The listing builds one solid part. Answer for the finished solid, in the listing's coordinates (mm). A direction names the side the tool comes from. Round coordinates to 2 decimals unless told otherwise and drop trailing zeros. Order: outer loops, then holes, each group sorted by start corner. A loop starts at its lowest first (then second) coordinate and runs counter-clockwise, first axis right, second up. Notation, with made-up numbers: M 87,51.25 L 92,51.25 A26 ccw 92,76.25 Z; hole C -28.5,-6.5 d11. An arc over 180 degrees is marked long. Write item = value, one per line. Start each with the question number.
(1) A cutting plane is placed at B-B, the plane y = 6.75. Determine the outline of the cut face in (x, z), and give its area (3 significant figures).
(2) A cutting plane is placed at C-C, the plane x = 0. Determine the outline of the cut face in (y, z).
(3) A cutting plane is placed at A-A, the plane x = 130. Determine the outline of the cut face in (y, z), and give its area (3 significant figures).
(4) Straight lines are drawn through the part: probe 1 along Z at (x, y) = (127, 3.25); probe 2 along X at (y, z) = (7, 0); probe 3 along Z at (x, y) = (220, 7). For each, find the intervals that lie inside material, in ascending order. Write a range as from..to.
(5) For a pull along X with two mould halves and no side action, classify faces 1 (the face through (193.228, 5.07, -4.797)), 2 (the face through (107, 10, 0)) as released by +X, released by -X, zero draft, split by the parting line, or undercut.
(6) Which of the six approach directions +Z, -Z, +X, -X, +Y, -Y give full straight-line access (tool end or side, diameter ignored) to faces 3 (the face through (29.369, 5, 0)), 4 (the face through (13.54, 5.07, -12.557)), 5 (the face through (210.5, 5.07, 12.35))?
(7) Each of these flat-tipped pins is pushed along its axis until it touches: pin 1 (4 mm diameter, centred on x = 98.5, y = 5.5, fed in from -Z); pin 2 (4 mm diameter, centred on y = 4.5, z = 9, fed in from -X); pin 3 (2 mm diameter, centred on x = 220, y = 2.5, fed in from -Z). Where does it stop, or does it pass through?
from build123d import *

# Parameters (mm, degrees)
SKETCH1_W           = 75
SKETCH1_H           = 12
SKETCH1_R           = 17.5
SKETCH1_R_2         = 11
SKETCH1_R_3         = 15
SKETCH1_R_4         = 8.75
BOSS_EXTRUDE1_DEPTH = 10
FILLET1_R           = 4
FILLET2_R           = 12
SKETCH2_R           = 1.25
CUT_EXTRUDE1_DEPTH  = 9


with BuildPart() as part:
    # Sketch1 → Boss-Extrude1 (new body)
    with BuildSketch(Plane(origin=(0, 0, 0), x_dir=(1, 0, 0), z_dir=(0, 1, 0))):
        with BuildLine():
            Line((211, 12), (12.737739203, 12))
            ThreePointArc((12.737739203, 12), (16.265921985, 6.45521355), (17.5, 0))
            ThreePointArc((17.5, 0), (16.265921985, -6.45521355), (12.737739203, -12))
            Line((12.737739203, -12), (211, -12))
            ThreePointArc((211, -12), (205, 0), (211, 12))
        make_face()
        with Locations((66.868869601, 0)):
            Rectangle(SKETCH1_W, SKETCH1_H, mode=Mode.SUBTRACT)
        with Locations((156.868869601, 0)):
            Rectangle(SKETCH1_W, SKETCH1_H, mode=Mode.SUBTRACT)
        Circle(SKETCH1_R)
        Circle(SKETCH1_R_2, mode=Mode.SUBTRACT)
        with Locations((220, 0)):
            Circle(SKETCH1_R_3)
        with Locations((220, 0)):
            Circle(SKETCH1_R_4, mode=Mode.SUBTRACT)
    extrude(amount=BOSS_EXTRUDE1_DEPTH)

    # Fillet1
    fillet1_edges = [part.edges().sort_by_distance(p)[0] for p in [
        (119.368869601, 5, -6),
        (119.368869601, 5, 6),
        (194.368869601, 5, 6),
        (194.368869601, 5, -6),
        (29.368869601, 5, -6),
        (29.368869601, 5, 6),
        (104.368869601, 5, 6),
        (104.368869601, 5, -6),
    ]]
    fillet(fillet1_edges, radius=FILLET1_R)

    # Fillet2
    fillet2_edges = [part.edges().sort_by_distance(p)[0] for p in [
        (12.737739203, 5, 12),
        (12.737739203, 5, -12),
        (211, 5, -12),
        (211, 5, 12),
    ]]
    fillet(fillet2_edges, radius=FILLET2_R)

    # Sketch2 → Cut-Extrude1 (cut, symmetric)
    with BuildSketch(Plane.XY.offset(12)):
        with Locations((220, 2.5)):
            Circle(SKETCH2_R)
    extrude(amount=CUT_EXTRUDE1_DEPTH, both=True, mode=Mode.SUBTRACT)


solid = part.part
Reported:
q1.outline = M 10.18,-14.24 A12 cw 17.15,-12 L 207.63,-12 A12 cw 213.13,-13.33 A15 ccw long 213.13,13.33 A12 cw 207.63,12 L 17.15,12 A12 cw 10.18,14.24 A17.5 ccw long Z; hole C 0,0 d22; hole M 29.37,-2 A4 ccw 33.37,-6 L 100.37,-6 A4 ccw 104.37,-2 L 104.37,2 A4 ccw 100.37,6 L 33.37,6 A4 ccw 29.37,2 Z; hole M 119.37,-2 A4 ccw 123.37,-6 L 190.37,-6 A4 ccw 194.37,-2 L 194.37,2 A4 ccw 190.37,6 L 123.37,6 A4 ccw 119.37,2 Z; hole C 220,0 d17.5
q1.area = 3,860 mm²
q2.outline = M 0,-17.5 L 10,-17.5 L 10,-11 L 0,-11 Z; M 0,11 L 10,11 L 10,17.5 L 0,17.5 Z
q3.outline = M 0,-12 L 10,-12 L 10,-6 L 0,-6 Z; M 0,6 L 10,6 L 10,12 L 0,12 Z
q3.area = 120 mm²
q4.probe_1 = -12..-6, 6..12
q4.probe_2 = -17.5..-11, 11..29.37, 104.37..119.37, 194.37..211.25, 228.75..235
q4.probe_3 = -15..-8.75, 8.75..15
q5.face_1 = undercut
q5.face_2 = zero draft
q6.face_3 = +Y, -Y
q6.face_4 = -Z, +Y, -Y
q6.face_5 = +Z, +Y, -Y
q7.pin_1 = -12
q7.pin_2 = -16.04
q7.pin_3 = -15
